Autodesk Inventor part; units mm, degrees
ref_plane "YZ Plane" through (0, 0, 0) normal (1, 0, 0) x (0, 1, 0)
ref_plane "XZ Plane" through (0, 0, 0) normal (0, 1, 0) x (-1, 0, 0)
ref_plane "XY Plane" through (0, 0, 0) normal (0, 0, 1) x (1, 0, 0)
sketch "Sketch1" plane through (0, 0, 0) normal (0, 0, 1) x (1, 0, 0)
  circle A0 centre (-194.945, 6.4301) radius 3.3782
  circle A1 centre (-194.945, 25.4801) radius 3.3782
  circle A2 centre (-144.145, 6.4301) radius 3.3782
  circle A3 centre (-144.145, 25.4801) radius 3.3782
  circle A4 centre (-169.545, 15.9551) radius 14.2875
  line L0 (-254, -1.8249) -> (254, -1.8249) construction
  line L1 (-247.65, 40.5304) -> (247.65, 40.5304) construction
  line L2 (-204.47, -0.5549) -> (-204.47, 32.4651)
  line L3 (-204.47, 32.4651) -> (-134.62, 32.4651)
  line L4 (-134.62, 32.4651) -> (-134.62, -0.5549)
  line L5 (-134.62, -0.5549) -> (-204.47, -0.5549)
  point P0 (0, 0)
extrude "Extrusion1" add sketch "Sketch1" along normal blind 3.175 contours A0 | A4 | L2 L3 L4 L5
fillet "Fillet1" radius 6.35 4 edges at (-204.47, 32.4651, 1.5875) (-204.47, -0.5549, 1.5875) (-134.62, 32.4651, 1.5875) (-134.62, -0.5549, 1.5875)
sketch "Sketch2" plane through (0, 0, 3.175) normal (0, 0, 1) x (1, 0, 0)
  line L0 (-134.62, 26.1151) -> (-134.62, 5.7951)
  line L1 (-198.12, 32.4651) -> (-140.97, 32.4651)
  line L2 (-204.47, 5.7951) -> (-204.47, 26.1151)
  line L3 (-140.97, -0.5549) -> (-198.12, -0.5549)
  line L4 (-169.545, 32.4651) -> (-169.545, -0.5549) construction
  line L5 (-204.47, 15.9551) -> (-134.62, 15.9551) construction
  circle A0 centre (-175.045, 24.9551) radius 1.3
  circle A1 centre (-164.045, 24.9551) radius 1.3
  circle A2 centre (-175.045, 6.9551) radius 1.3
  circle A3 centre (-164.045, 6.9551) radius 1.3
  line L6 (-175.045, 24.9551) -> (-164.045, 24.9551) construction
  line L7 (-175.045, 6.9551) -> (-164.045, 6.9551) construction
  line L8 (-175.045, 24.9551) -> (-175.045, 6.9551) construction
  line L9 (-165.545, 21.9551) -> (-165.545, 9.9551)
  line L10 (-165.545, 9.9551) -> (-162.045, 9.9551)
  line L11 (-162.045, 9.9551) -> (-162.045, 21.9551)
  line L12 (-162.045, 21.9551) -> (-165.545, 21.9551)
  circle A4 centre (-187.545, 8.9551) radius 5
  point P0 (0, 0)
  point P1 (-169.545, 6.9551)
  point P2 (-175.045, 15.9551)
  point P3 (-162.045, 15.9551)
  dimension "d7" = 2.6
  dimension "d10" = 11
  dimension "d13" = 18
  dimension "d16" = 12
  dimension "d17" = 3.5
  dimension "d18" = 4
  dimension "d19" = 10
  dimension "d20" = 7
  dimension "d21" = 18
extrude "Extrusion2" cut sketch "Sketch2" against normal through all
equation "\"d2\" = d1"
properties part number "V5 Shooter Bearing Encoder Plate" material "Polycarbonate, Clear"
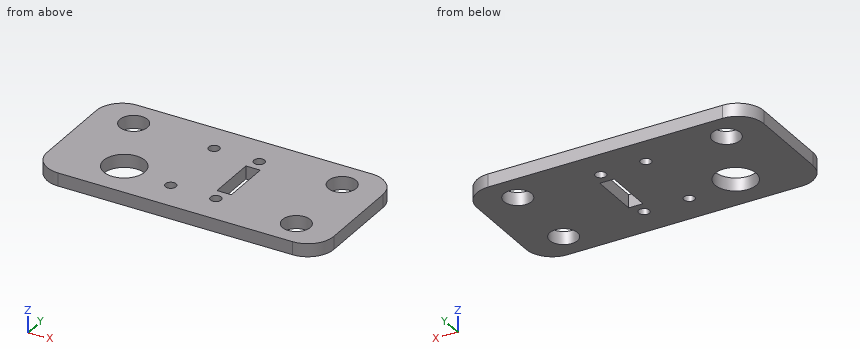
Verification items for the finished model (mm, model axes). Give positions to 0.01 mm unless a question says otherwise; leave off trailing zeros. Order: outer loops, then holes, each group sorted by start corner. A loop starts at its lowest first (then second) coordinate and runs counter-clockwise, first axis right, second up. Notation, with made-up numbers: M 42,-7 L 92,-7 A31 cw 92,25 Z; hole C 86,58.5 d8. An arc over 180 degrees is marked long. Answer in a Markdown table with one row per item. Add a question column.
Item 1: Section check C-C, the plane y = 23. Enter the section's corners in (x, z) (3 decimals), and give its area (3 significant figures).
Item 2: Section check A-A, the plane y = 19.5. Enter the section's corners in (x, z) (3 decimals).
Item 3: Scan lines: probe 1 along X at (y, z) = (4.5, 0.6); probe 2 along X at (y, z) = (20, 1.6) (3 decimals); probe 3 along Y at (x, z) = (-174, 0.2). Record each from-to range of solid material in increasing order. Write a range as from..to.
Item 4: Section check B-B, the plane z = 1.6. State how many separate pieces and enclosed holes the cut face has, and give its area (3 significant figures).
Item 5: Gauge pin test, flat end, axial feed: pin 1 (8 mm diameter, centred on x = -187.54, y = 8.96, fed in from +Z). Record the tip position at first contact, or that the pin passes through.
Filled sheet:
| question | item | result |
|---|---|---|
| 1 | outline | M -204.47,0 L -197.239,0 L -197.239,3.175 L -204.47,3.175 Z; M -192.651,0 L -146.439,0 L -146.439,3.175 L -192.651,3.175 Z; M -141.851,0 L -134.62,0 L -134.62,3.175 L -141.851,3.175 Z |
| 1 | area | 193 mm^2 |
| 2 | outline | M -204.47,0 L -165.545,0 L -165.545,3.175 L -204.47,3.175 Z; M -162.045,0 L -134.62,0 L -134.62,3.175 L -162.045,3.175 Z |
| 3 | probe 1 | x = -204.34..-189.81, -185.28..-146.92, -141.37..-134.75 |
| 3 | probe 2 | x = -204.47..-165.545, -162.045..-134.62 |
| 3 | probe 3 | y = -0.55..6.18, 7.73..24.18, 25.73..32.47 |
| 4 | separate pieces | 1 |
| 4 | enclosed holes | 9 |
| 4 | area | 2,020 mm^2 |
| 5 | pin 1 | passes through |
